Autodesk Inventor part; units mm, degrees
ref_plane "YZ Plane" through (0, 0, 0) normal (1, 0, 0) x (0, 1, 0)
ref_plane "XZ Plane" through (0, 0, 0) normal (0, 1, 0) x (-1, 0, 0)
ref_plane "XY Plane" through (0, 0, 0) normal (0, 0, 1) x (1, 0, 0)
sketch "Sketch1" plane through (0, 0, 0) normal (0, 0, 1) x (1, 0, 0)
  line L0 (0, 0) -> (152.4, 0)
  line L1 (152.4, 0) -> (152.4, -152.4)
  line L2 (152.4, -152.4) -> (0, -152.4)
  line L3 (0, -152.4) -> (0, 0)
  line L4 (0, -152.4) -> (-50.8, -152.4) construction
  line L5 (-50.8, -152.4) -> (-50.8, 25.4) construction
  line L6 (0, 0) -> (0, -152.4)
  line L7 (-47.625, 25.4) -> (152.4, 25.4) construction
  line L8 (152.4, 25.4) -> (152.4, 0) construction
  line L9 (152.4, 0) -> (0, 0)
  line L10 (-47.625, 0) -> (-47.625, 25.4) construction
  line L11 (-50.8, -152.4) -> (-50.8, 25.4) construction
  line L12 (-50.8, 25.4) -> (-47.625, 25.4) construction
  circle A0 centre (60.96, -60.96) radius 54.61 construction
  circle A1 centre (60.96, -60.96) radius 53.34 construction
  circle A2 centre (60.96, -60.96) radius 17.4625
  line L13 (0, 0) -> (-47.625, 0) construction
  line L14 (0, -152.4) -> (-9.525, -152.4)
  line L15 (-9.525, -152.4) -> (-9.525, 3.175)
  line L16 (-3.175, 9.525) -> (152.4, 9.525)
  line L17 (152.4, 0) -> (152.4, 9.525)
  circle A3 centre (60.96, -60.96) radius 47.2059 construction
  line L18 (-4.7625, 9.525) -> (-4.7625, -152.4) construction
  line L19 (-9.525, 4.7625) -> (152.4, 4.7625) construction
  arc A4 (-3.175, 9.525) -> (-9.525, 3.175) centre (-3.175, 3.175) ccw
  point P0 (-9.525, 9.525)
  point P1 (12.7, 4.7625)
  point P2 (-4.7625, -12.7)
  point P3 (76.2, 4.7625)
  point P4 (139.7, 4.7625)
  point P5 (-4.7625, -76.2)
  point P6 (-4.7625, -139.7)
  dimension "d0" = 152.4
  dimension "d8" = 50.8
  dimension "d12" = 3.175
  dimension "d28" = 152.4
  dimension "d29" = 109.22
  dimension "d30" = 106.68
  dimension "d31" = 60.96
  dimension "d32" = 60.96
  dimension "d33" = 34.925
  dimension "d34" = 9.525
  dimension "d35" = 9.525
  dimension "d41" = 94.4118
  dimension "d42" = 25.4
  dimension "d43" = 22.225
  dimension "d44" = 22.225
  dimension "d45" = 6.35
  dimension "d48" = 63.5
  dimension "d55" = 63.5
extrude "Extrusion1" add sketch "Sketch1" along normal blind 4.7625
hole "Hole1" at (12.7, 4.7625, 0) at (-4.7625, -12.7, 0) at (76.2, 4.7625, 0) at (139.7, 4.7625, 0) at (-4.7625, -76.2, 0) at (-4.7625, -139.7, 0) direction (0, 0, 1) diameter 4.9784 end through all
properties part number "Module Plate - Bottom"
The listing builds one solid part. Answer for the finished solid, in the listing's coordinates (mm). Round coordinates to 2 decimals unless told otherwise and drop trailing zeros. Loops run counter-clockwise (first coordinate to the right, second up) from the corner with the lowest first, then second, coordinate; pieces in that order, holes last. Notation, with made-up numbers: (-6, -32) - (35, -32) arc R5 cw to (35, -24) - close; hole circle Ø10 at (-13.5, 14). An arc over 180 degrees is marked (long way). Use one line per item in the form item = value. Start each with the question number.
1. Consider line 1 (X direction, y = -139.7, z = 3.7) (3 decimals); line 2 (Y direction, x = 60.96, z = 3.05) (1 decimal); line 3 (Y direction, x = 76.2, z = 2.95) (3 decimals). Determine where each line is inside the solid, lowest interval first. Write a range as [from, to].
2. The part is cut by section D-D on z = 2.7. Give the number of separate pieces and of enclosed holes in the cut face, then the cut area to 3 significant figures.
3. The part is cut by section B-B on x = 12.7. Determine the outline of the cut face in (y, z) (1 decimal).
4. The part is cut by section C-C on x = 76.2. Determine the outline of the cut face in (y, z) (1 decimal).
5. For a pull along X with two mould halves and no side action, classify faces 1 (the face through (-7.71, 7.62, 2.35)), 2 (the face through (10.6, 6.1, 2.4)), 3 (the face through (88, -70, 4.762)) as pulls with the +X half, pulls with the -X half, needs draft (parallel to the pull), parting line crosses it, or undercut.
6. The part is cut by section A-A on y = -60.96. Determine the outline of the cut face in (x, z) (1 decimal), then the cut area to 3 significant figures.
Geometry check:
q1.line_1 = [-9.525, -7.252], [-2.273, 152.4]
q1.line_2 = [-152.4, -78.4], [-43.5, 9.5]
q1.line_3 = [-152.4, -69.485], [-52.435, 2.273], [7.252, 9.525]
q2.separate_pieces = 1
q2.enclosed_holes = 7
q2.area = 25,100 mm^2
q3.outline = (-152.4, 0) - (2.3, 0) - (2.3, 4.8) - (-152.4, 4.8) - close; (7.3, 0) - (9.5, 0) - (9.5, 4.8) - (7.3, 4.8) - close
q4.outline = (-152.4, 0) - (-69.5, 0) - (-69.5, 4.8) - (-152.4, 4.8) - close; (-52.4, 0) - (2.3, 0) - (2.3, 4.8) - (-52.4, 4.8) - close; (7.3, 0) - (9.5, 0) - (9.5, 4.8) - (7.3, 4.8) - close
q5.face_1 = pulls with the -X half
q5.face_2 = undercut
q5.face_3 = needs draft
q6.outline = (-9.5, 0) - (43.5, 0) - (43.5, 4.8) - (-9.5, 4.8) - close; (78.4, 0) - (152.4, 0) - (152.4, 4.8) - (78.4, 4.8) - close
q6.area = 605 mm^2
